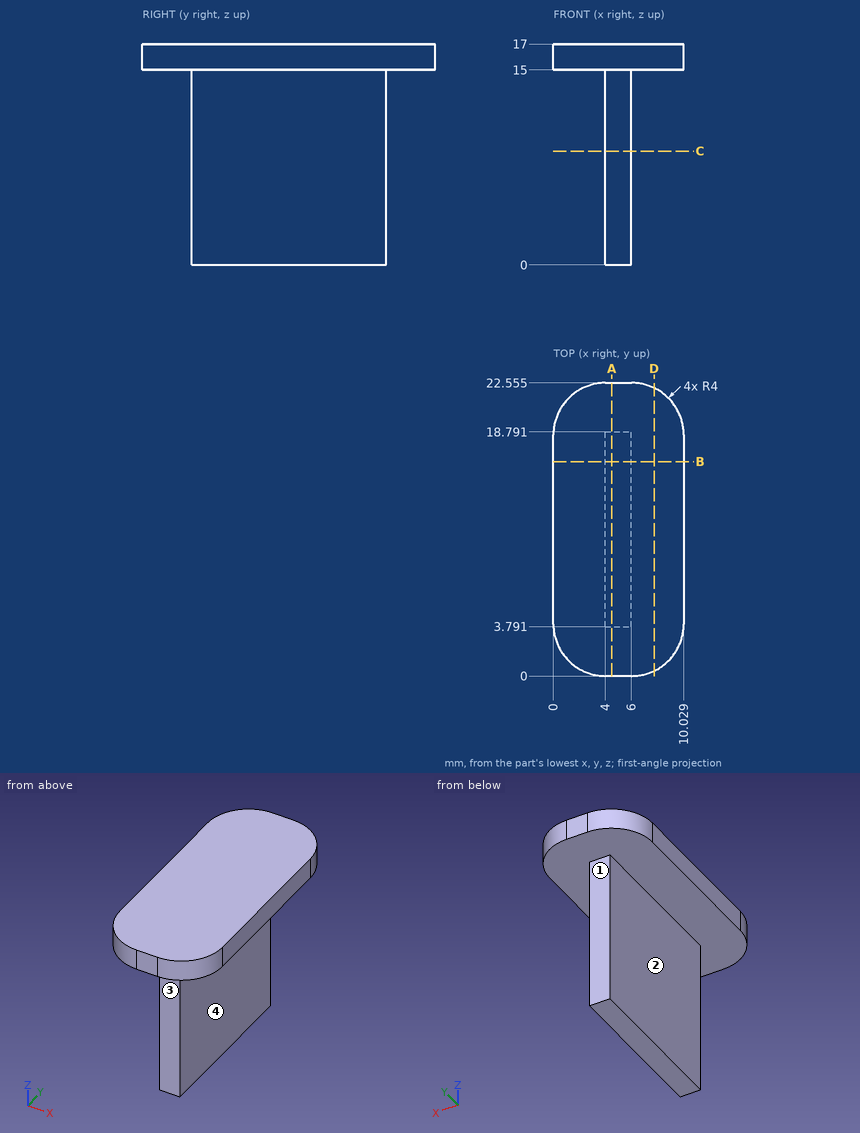
Study the drawing (mm; zero at the part's minimum x, y, z) and answer. A direction names the side the tool comes from. Give positions to 0.01 mm unless a question says otherwise; leave off trailing zeros. Write each loop counter-clockwise with the first axis right and the second up, starting at its lowest first coordinate (ties: lowest second). Pieces come first, ordered by that corner, then holes.
Item 1: Find the intervals of material crossed by line 1 along Y through (x, z) = (4.5, 7.75); line 2 along X through (y, z) = (18, 11.5); line 3 along Z through (x, y) = (5.25, 3.75), in increasing order.
Item 2: Section D-D, the plane x = 7.75 is taken. Write down the section's boundary in (y, z).
Item 3: Section B-B, the plane y = 16.5 is taken. Write down the section's boundary in (x, z).
Item 4: Section A-A, the plane x = 4.5 is taken. Write down the section's boundary in (y, z) (1 decimal), plus the area to 3 significant figures.
Item 5: Which of the six approach directions +Z, -Z, +X, -X, +Y, -Y give full straight-line access (tool end or side, diameter ignored) to the marked faces 1, 2, 3 and 4?
Item 6: Section C-C, the plane z = 8.75 is taken. Write down the section's boundary in (x, y), plus the area to 3 significant figures.
Item 7: Flat-ended cylindrical pins translate along their axes: P1, Ø7.5, axis at y = 8.5, z = 6.5, coming from the -X side; P2, Ø1.5, axis at y = 16.5, z = 5, coming from the +X side; P3, Ø3, axis at x = 5.5, z = 3, coming from the +Y side. Find the tip coordinate at first contact, or state that the pin passes through.
Completed:
1. line 1: y = 3.79 to 18.79
1. line 2: x = 4 to 6
1. line 3: z = 15 to 17
2. outline: (0.39, 15) - (22.17, 15) - (22.17, 17) - (0.39, 17) - close
3. outline: (0, 15) - (4, 15) - (4, 0) - (6, 0) - (6, 15) - (10.03, 15) - (10.03, 17) - (0, 17) - close
4. outline: (0, 15) - (3.8, 15) - (3.8, 0) - (18.8, 0) - (18.8, 15) - (22.6, 15) - (22.6, 17) - (0, 17) - close
4. area: 270 mm2
5. face 1: -Z, +X, -X, +Y
5. face 2: -Z, -X, +Y, -Y
5. face 3: -Z, +X, -X, -Y
5. face 4: -Z, +X, +Y, -Y
6. outline: (4, 3.79) - (6, 3.79) - (6, 18.79) - (4, 18.79) - close
6. area: 30.0 mm2
7. P1: stops at x = 4
7. P2: stops at x = 6
7. P3: stops at y = 18.79
